```python
from build123d import *

# Parameters (mm, degrees)
CROQUIS1_R              = 1.75
SALIENTE_EXTRUIR1_DEPTH = 8


with BuildPart() as part:
    # Croquis1 → Saliente-Extruir1 (new body)
    with BuildSketch(Plane(origin=(0, 0, 0), x_dir=(1, 0, 0), z_dir=(0, 1, 0))):
        with BuildLine():
            ThreePointArc((26.318983455, 14.228225469), (34.708358258, 66.001642936), (87.111019212, 63.804032696))
            Line((87.111019212, 63.804032696), (91.223264764, 67.638763711))
            Line((91.223264764, 67.638763711), (91.448573923, 70.544764206))
            ThreePointArc((91.448573923, 70.544764206), (30.189185372, 72.489467715), (18.249404228, 12.373445028))
            Line((18.249404228, 12.373445028), (9.60277667, 7.349917196))
            ThreePointArc((9.60277667, 7.349917196), (8.915528014, 8.169942644), (8.158486898, 8.926012217))
            ThreePointArc((8.158486898, 8.926012217), (8.809805691, 10.105820521), (9.148703928, 11.410163953))
            ThreePointArc((9.148703928, 11.410163953), (8.903135899, 11.602792602), (8.65351323, 11.79013714))
            ThreePointArc((8.65351323, 11.79013714), (7.48132754, 11.125197659), (6.510293938, 10.190715157))
            ThreePointArc((6.510293938, 10.190715157), (6.046375, 10.472628702), (5.57027124, 10.733437515))
            ThreePointArc((5.57027124, 10.733437515), (5.894040025, 12.041618533), (5.883801663, 13.389230859))
            ThreePointArc((5.883801663, 13.389230859), (5.596745198, 13.511738163), (5.30713988, 13.62809199))
            ThreePointArc((5.30713988, 13.62809199), (4.382711316, 12.654251603), (3.650909885, 11.528463019))
            ThreePointArc((3.650909885, 11.528463019), (3.129834008, 11.680699536), (2.602450802, 11.809396783))
            ThreePointArc((2.602450802, 11.809396783), (2.576605271, 13.156800143), (2.217928037, 14.455843809))
            ThreePointArc((2.217928037, 14.455843809), (1.908945561, 14.499881098), (1.599093719, 14.537314892))
            ThreePointArc((1.599093719, 14.537314892), (0.916420874, 13.375367565), (0.542722358, 12.080565177))
            ThreePointArc((0.542722358, 12.080565177), (0, 12.09275), (-0.542722358, 12.080565177))
            ThreePointArc((-0.542722358, 12.080565177), (-0.916420874, 13.375367565), (-1.599093719, 14.537314892))
            ThreePointArc((-1.599093719, 14.537314892), (-1.908945561, 14.499881098), (-2.217928037, 14.455843809))
            ThreePointArc((-2.217928037, 14.455843809), (-2.576605271, 13.156800143), (-2.602450802, 11.809396783))
            ThreePointArc((-2.602450802, 11.809396783), (-3.129834008, 11.680699536), (-3.650909885, 11.528463019))
            ThreePointArc((-3.650909885, 11.528463019), (-4.346994451, 12.682425791), (-5.30713988, 13.62809199))
            ThreePointArc((-5.30713988, 13.62809199), (-5.596745198, 13.511738163), (-5.883801663, 13.389230859))
            ThreePointArc((-5.883801663, 13.389230859), (-5.894040025, 12.041618533), (-5.57027124, 10.733437515))
            ThreePointArc((-5.57027124, 10.733437515), (-6.046375, 10.472628702), (-6.510293938, 10.190715157))
            ThreePointArc((-6.510293938, 10.190715157), (-7.48132754, 11.125197659), (-8.65351323, 11.79013714))
            ThreePointArc((-8.65351323, 11.79013714), (-8.903135899, 11.602792602), (-9.148703928, 11.410163953))
            ThreePointArc((-9.148703928, 11.410163953), (-8.809805691, 10.105820521), (-8.158486898, 8.926012217))
            ThreePointArc((-8.158486898, 8.926012217), (-8.550865528, 8.550865528), (-8.926012217, 8.158486898))
            ThreePointArc((-8.926012217, 8.158486898), (-10.105820521, 8.809805691), (-11.410163953, 9.148703928))
            ThreePointArc((-11.410163953, 9.148703928), (-11.602792602, 8.903135899), (-11.79013714, 8.65351323))
            ThreePointArc((-11.79013714, 8.65351323), (-11.125197659, 7.48132754), (-10.190715157, 6.510293938))
            ThreePointArc((-10.190715157, 6.510293938), (-10.472628702, 6.046375), (-10.733437515, 5.57027124))
            ThreePointArc((-10.733437515, 5.57027124), (-12.041618533, 5.894040025), (-13.389230859, 5.883801663))
            ThreePointArc((-13.389230859, 5.883801663), (-13.511738163, 5.596745198), (-13.62809199, 5.30713988))
            ThreePointArc((-13.62809199, 5.30713988), (-12.682425791, 4.346994451), (-11.528463019, 3.650909885))
            ThreePointArc((-11.528463019, 3.650909885), (-11.680699536, 3.129834008), (-11.809396783, 2.602450802))
            ThreePointArc((-11.809396783, 2.602450802), (-13.156800143, 2.576605271), (-14.455843809, 2.217928037))
            ThreePointArc((-14.455843809, 2.217928037), (-14.499881098, 1.908945561), (-14.537314892, 1.599093719))
            ThreePointArc((-14.537314892, 1.599093719), (-13.375367565, 0.916420874), (-12.080565177, 0.542722358))
            ThreePointArc((-12.080565177, 0.542722358), (-12.09275, 0), (-12.080565177, -0.542722358))
            ThreePointArc((-12.080565177, -0.542722358), (-13.375367565, -0.916420874), (-14.537314892, -1.599093719))
            ThreePointArc((-14.537314892, -1.599093719), (-14.499881098, -1.908945561), (-14.455843809, -2.217928037))
            ThreePointArc((-14.455843809, -2.217928037), (-13.156800143, -2.576605271), (-11.809396783, -2.602450802))
            ThreePointArc((-11.809396783, -2.602450802), (-11.680699536, -3.129834008), (-11.528463019, -3.650909885))
            ThreePointArc((-11.528463019, -3.650909885), (-12.682425791, -4.346994451), (-13.62809199, -5.30713988))
            ThreePointArc((-13.62809199, -5.30713988), (-13.511738163, -5.596745198), (-13.389230859, -5.883801663))
            ThreePointArc((-13.389230859, -5.883801663), (-12.041618533, -5.894040025), (-10.733437515, -5.57027124))
            ThreePointArc((-10.733437515, -5.57027124), (-10.472628702, -6.046375), (-10.190715157, -6.510293938))
            ThreePointArc((-10.190715157, -6.510293938), (-11.125197659, -7.48132754), (-11.79013714, -8.65351323))
            ThreePointArc((-11.79013714, -8.65351323), (-11.602792602, -8.903135899), (-11.410163953, -9.148703928))
            ThreePointArc((-11.410163953, -9.148703928), (-10.105820521, -8.809805691), (-8.926012217, -8.158486898))
            ThreePointArc((-8.926012217, -8.158486898), (-8.550865528, -8.550865528), (-8.158486898, -8.926012217))
            ThreePointArc((-8.158486898, -8.926012217), (-8.809805691, -10.105820521), (-9.148703928, -11.410163953))
            ThreePointArc((-9.148703928, -11.410163953), (-8.903135899, -11.602792602), (-8.65351323, -11.79013714))
            ThreePointArc((-8.65351323, -11.79013714), (-7.48132754, -11.125197659), (-6.510293938, -10.190715157))
            ThreePointArc((-6.510293938, -10.190715157), (-6.046375, -10.472628702), (-5.57027124, -10.733437515))
            ThreePointArc((-5.57027124, -10.733437515), (-5.894040025, -12.041618533), (-5.883801663, -13.389230859))
            ThreePointArc((-5.883801663, -13.389230859), (-5.596745198, -13.511738163), (-5.30713988, -13.62809199))
            ThreePointArc((-5.30713988, -13.62809199), (-4.346994451, -12.682425791), (-3.650909885, -11.528463019))
            ThreePointArc((-3.650909885, -11.528463019), (-3.129834008, -11.680699536), (-2.602450802, -11.809396783))
            ThreePointArc((-2.602450802, -11.809396783), (-2.576605271, -13.156800143), (-2.217928037, -14.455843809))
            ThreePointArc((-2.217928037, -14.455843809), (-1.908945561, -14.499881098), (-1.599093719, -14.537314892))
            ThreePointArc((-1.599093719, -14.537314892), (-0.916420874, -13.375367565), (-0.542722358, -12.080565177))
            ThreePointArc((-0.542722358, -12.080565177), (0, -12.09275), (0.542722358, -12.080565177))
            ThreePointArc((0.542722358, -12.080565177), (0.916420874, -13.375367565), (1.599093719, -14.537314892))
            ThreePointArc((1.599093719, -14.537314892), (1.908945561, -14.499881098), (2.217928037, -14.455843809))
            ThreePointArc((2.217928037, -14.455843809), (2.576605271, -13.156800143), (2.602450802, -11.809396783))
            ThreePointArc((2.602450802, -11.809396783), (3.129834008, -11.680699536), (3.650909885, -11.528463019))
            ThreePointArc((3.650909885, -11.528463019), (4.346994451, -12.682425791), (5.30713988, -13.62809199))
            ThreePointArc((5.30713988, -13.62809199), (5.596745198, -13.511738163), (5.883801663, -13.389230859))
            ThreePointArc((5.883801663, -13.389230859), (5.894040025, -12.041618533), (5.57027124, -10.733437515))
            ThreePointArc((5.57027124, -10.733437515), (6.046375, -10.472628702), (6.510293938, -10.190715157))
            ThreePointArc((6.510293938, -10.190715157), (7.48132754, -11.125197659), (8.65351323, -11.79013714))
            ThreePointArc((8.65351323, -11.79013714), (8.903135899, -11.602792602), (9.148703928, -11.410163953))
            ThreePointArc((9.148703928, -11.410163953), (8.809805691, -10.105820521), (8.158486898, -8.926012217))
            ThreePointArc((8.158486898, -8.926012217), (8.550865528, -8.550865528), (8.926012217, -8.158486898))
            ThreePointArc((8.926012217, -8.158486898), (10.105820521, -8.809805691), (11.410163953, -9.148703928))
            ThreePointArc((11.410163953, -9.148703928), (11.602792602, -8.903135899), (11.79013714, -8.65351323))
            ThreePointArc((11.79013714, -8.65351323), (11.125197659, -7.48132754), (10.190715157, -6.510293938))
            ThreePointArc((10.190715157, -6.510293938), (10.472628702, -6.046375), (10.733437515, -5.57027124))
            ThreePointArc((10.733437515, -5.57027124), (11.748007896, -2.866864669), (12.09275, 0))
            Line((12.09275, 0), (24.597080908, 7.219378816))
            ThreePointArc((24.597080908, 7.219378816), (26.952693775, 10.356600271), (26.318983455, 14.228225469))
        make_face()
        with Locations(Location((0, 0, 0), (0, 0, 270))):
            Circle(CROQUIS1_R, mode=Mode.SUBTRACT)
    extrude(amount=SALIENTE_EXTRUIR1_DEPTH)


solid = part.part
```
Design review of the part built by this model. Coordinates are the model's own, in mm. A direction names the side the tool comes from. Coordinates: 2 decimals unless noted, no trailing zeros. Order: outer loops, then holes, each group sorted by start corner. A loop starts at its lowest first (then second) coordinate and runs counter-clockwise, first axis right, second up.
1) Wall thickness on line 1 along X through (y, z) = (3.25, 0); line 2 along X through (y, z) = (5, -12); line 3 along X through (y, z) = (1, -68): over which ranges is each line inside the solid? List them lowest first.
2) Mouldability with a two-part tool opening along X and no side actions: class faces 5 (the cylindrical face through (-13.393, 3.944, -0.924)), 6 (the cylindrical face through (-12.02, 3.94, -5.89)), 7 (the flat face through (91.334, 3.944, -69.071)), 8 (the flat face through (19, 8, -34)) as +X half, -X half, draft (parallel to the pull), parting line (faces both ways), or undercut.
3) For faces 1 (the cylindrical face through (8.803, 3.944, -10.088)), 2 (the cylindrical face through (-13.36, 3.94, 0.91)), 3 (the cylindrical face through (-0.924, 3.944, 13.393)), 4 (the cylindrical face through (0.924, 3.944, -13.393)), list the 3-axis set-ups (+Z, -Z, +X, -X, +Y, -Y) from which the entire face can be reached by the end or side of a thin tool; tool diameter is ignored.
4) Take a section at B-B, the plane z = -50.5. Give the boundary of the cut face in (x, y).
5) Take a section at A-A, the plane x = 41.5. Give the boundary of the cut face in (y, z), and give its area (3 significant figures).
6) Clearance check with flat-ended pins moving along their axes: pin 1 (3 mm diameter, centred on y = 4, z = -20, fed in from +X); pin 2 (3 mm diameter, centred on y = 3.5, z = -18, fed in from +X); pin 3 (2 mm diameter, centred on x = 24.5, y = 2, fed in from +Z). State where each tip first meets the part, or that it passes through.
Returned:
1. line 1: x = -12.09 to -1.75, 1.75 to 12.09
1. line 2: x = -5.89 to -3.89, -2.62 to 2.62, 3.92 to 5.89, 17.61 to 27.08
1. line 3: x = 25.29 to 37.38, 81.96 to 91.25
2. face 5: -X half
2. face 6: undercut
2. face 7: +X half
2. face 8: draft
3. face 1: +Y, -Y
3. face 2: -X, +Y, -Y
3. face 3: +Z, +Y, -Y
3. face 4: -Z, +Y, -Y
4. outline: (14.76, 0) - (23.18, 0) - (23.18, 8) - (14.76, 8) - close
5. outline: (0, -79.16) - (8, -79.16) - (8, -70.46) - (0, -70.46) - close
5. area: 69.5 mm2
6. pin 1: stops at x = 23.97
6. pin 2: stops at x = 24.98
6. pin 3: stops at z = -6.59
